Here's how the part is built. I have some questions about the finished solid (model axes, mm). Coordinates: 2 decimals unless noted, no trailing zeros. Write each loop counter-clockwise with the first axis right and the second up, starting at its lowest first coordinate (ties: lowest second). Pieces come first, ordered by that corner, then holes. Notation, with made-up numbers: M 26.25,47.5 L 54.25,47.5 A27 ccw 54.25,86.5 Z; hole C -15,51 d8. An arc over 180 degrees is marked long. Use a Markdown table: item, result.
```python
from build123d import *

# Parameters (mm, degrees)
SKETCH2_W          = 50
SKETCH2_H          = 100
BASE_FLANGE1_DEPTH = 0.9
EDGE_FLANGE1_DEPTH = 100
SKETCH10_W         = 49.533692342
SKETCH10_H         = 24
CUT_EXTRUDE1_DEPTH = 10
SKETCH12_W         = 49.533692342
SKETCH12_H         = 24
CUT_EXTRUDE2_DEPTH = 10
SKETCH13_W         = 49.533692342
SKETCH13_H         = 24
CUT_EXTRUDE3_DEPTH = 10
SKETCH17_W         = 80
SKETCH17_H         = 20
TAB4_DEPTH         = 0.9


# Sheet-metal steps are written as plain solids
with BuildPart() as part:
    # Sketch2 → Base-Flange1 (new body)
    with BuildSketch(Plane.XY):
        Rectangle(SKETCH2_W, SKETCH2_H)
    extrude(amount=-BASE_FLANGE1_DEPTH)

    # Edge-Flange1 section (across the edge) → Edge-Flange1 (add)
    with BuildSketch(Plane(origin=(25.466307658, -50, 0), x_dir=(-0.7660444431189747, 0, 0.6427876096865435), z_dir=(0, 1, 0))):
        with BuildLine():
            Line((-0.9, 0.466307658), (-0.9, 50))
            Line((-0.9, 50), (0, 50))
            Line((0, 50), (0, 0.466307658))
            ThreePointArc((0, 0.466307658), (0.093692213, 0.043689396), (0.35721239, -0.299736785))
            Line((0.35721239, -0.299736785), (-0.221296458, -0.989176784))
            ThreePointArc((-0.221296458, -0.989176784), (-0.721984795, -0.336667039), (-0.9, 0.466307658))
        make_face()
    extrude(amount=EDGE_FLANGE1_DEPTH)

    # Sketch10 → Cut-Extrude1 (cut)
    with BuildSketch(Plane(origin=(14.944242787, 0, -12.539708611), x_dir=(0.6427876096865437, 0, 0.7660444431189746), z_dir=(-0.7660444431189746, 0, 0.6427876096865437))):
        with Locations((41.602580856, 38)):
            Rectangle(SKETCH10_W, SKETCH10_H)
    extrude(amount=-CUT_EXTRUDE1_DEPTH, mode=Mode.SUBTRACT)

    # Sketch12 → Cut-Extrude2 (cut)
    with BuildSketch(Plane(origin=(14.944242787, 0, -12.539708611), x_dir=(0.6427876096865437, 0, 0.7660444431189746), z_dir=(-0.7660444431189746, 0, 0.6427876096865437))):
        with Locations((41.602580856, 0)):
            Rectangle(SKETCH12_W, SKETCH12_H)
    extrude(amount=-CUT_EXTRUDE2_DEPTH, mode=Mode.SUBTRACT)

    # Sketch13 → Cut-Extrude3 (cut)
    with BuildSketch(Plane(origin=(14.944242787, 0, -12.539708611), x_dir=(0.6427876096865437, 0, 0.7660444431189746), z_dir=(-0.7660444431189746, 0, 0.6427876096865437))):
        with Locations((41.602580856, -38)):
            Rectangle(SKETCH13_W, SKETCH13_H)
    extrude(amount=-CUT_EXTRUDE3_DEPTH, mode=Mode.SUBTRACT)

    # Sketch17 → Tab4 (add)
    with BuildSketch(Plane.XY):
        with Locations((-25, 0)):
            Rectangle(SKETCH17_W, SKETCH17_H)
    extrude(amount=-TAB4_DEPTH)


solid = part.part
```
1. We'd pull the mould along Y, two halves only. Please class faces 1 (the face through (42, 12, 19)), 2 (the face through (42, -26, 19)), 3 (the face through (-1, 1, 0)): +Y half, -Y half, draft (parallel to the pull), parting line (faces both ways), or undercut.
Answers follow:
| item | result |
|---|---|
| face 1 | undercut |
| face 2 | -Y half |
| face 3 | draft |
2. Suppose I cut it at C-C on z = 2.5. Write out the boundary of the cut face in (x, y), and give its area (3 significant figures).
Answers follow:
| item | result |
|---|---|
| outline | M 27.56,-26 L 28.74,-26 L 28.74,-12 L 27.56,-12 Z; M 27.56,12 L 28.74,12 L 28.74,26 L 27.56,26 Z |
| area | 32.9 mm2 |
3. Suppose I cut it at D-D on x = -52.5. Write out the boundary of the cut face in (y, z).
Answers follow:
| item | result |
|---|---|
| outline | M -10,-0.9 L 10,-0.9 L 10,0 L -10,0 Z |
4. Will these pins go through, and if not, where does the flat tip stop? pin 1 Ø5 at (y, z) = (-15.5, 14.5) entering from -X; pin 2 Ø10 at (x, z) = (34.5, 15.5) entering from -Y; pin 3 Ø8 at (y, z) = (-4.5, 18) entering from -X; pin 4 Ø1 at (x, y) = (17.5, 20.5) entering from +Z.
Answers follow:
| item | result |
|---|---|
| pin 1 | stops at x = 35.54 |
| pin 2 | stops at y = -26 |
| pin 3 | passes through |
| pin 4 | stops at z = 0 |
5. Suppose I cut it at A-A on x = 28. Write out the boundary of the cut face in (y, z), and give its area (3 significant figures).
Answers follow:
| item | result |
|---|---|
| outline | M -26,1.62 L -12,1.62 L -12,3.02 L -26,3.02 Z; M 12,1.62 L 26,1.62 L 26,3.02 L 12,3.02 Z |
| area | 39.2 mm2 |
6. Suppose I cut it at B-B on y = -22. Write out the boundary of the cut face in (x, z), and give its area (3 significant figures).
Answers follow:
| item | result |
|---|---|
| outline | M -25,-0.9 L 25,-0.9 A1.9 ccw 26.46,-0.22 L 58.3,37.72 L 57.61,38.3 L 25.77,0.36 A1 cw 25,0 L -25,0 Z |
| area | 90.7 mm2 |
7. I need wall thicknesses on probe 1 along Z at (x, y) = (24, -14); probe 2 along X at (y, z) = (-23, 11); probe 3 along Z at (x, y) = (42, -14.5). Which ranges of each line are inside material? Lowest first, please.
Answers follow:
| item | result |
|---|---|
| probe 1 | z = -0.9 to 0 |
| probe 2 | x = 34.7 to 35.87 |
| probe 3 | z = 18.3 to 19.7 |
